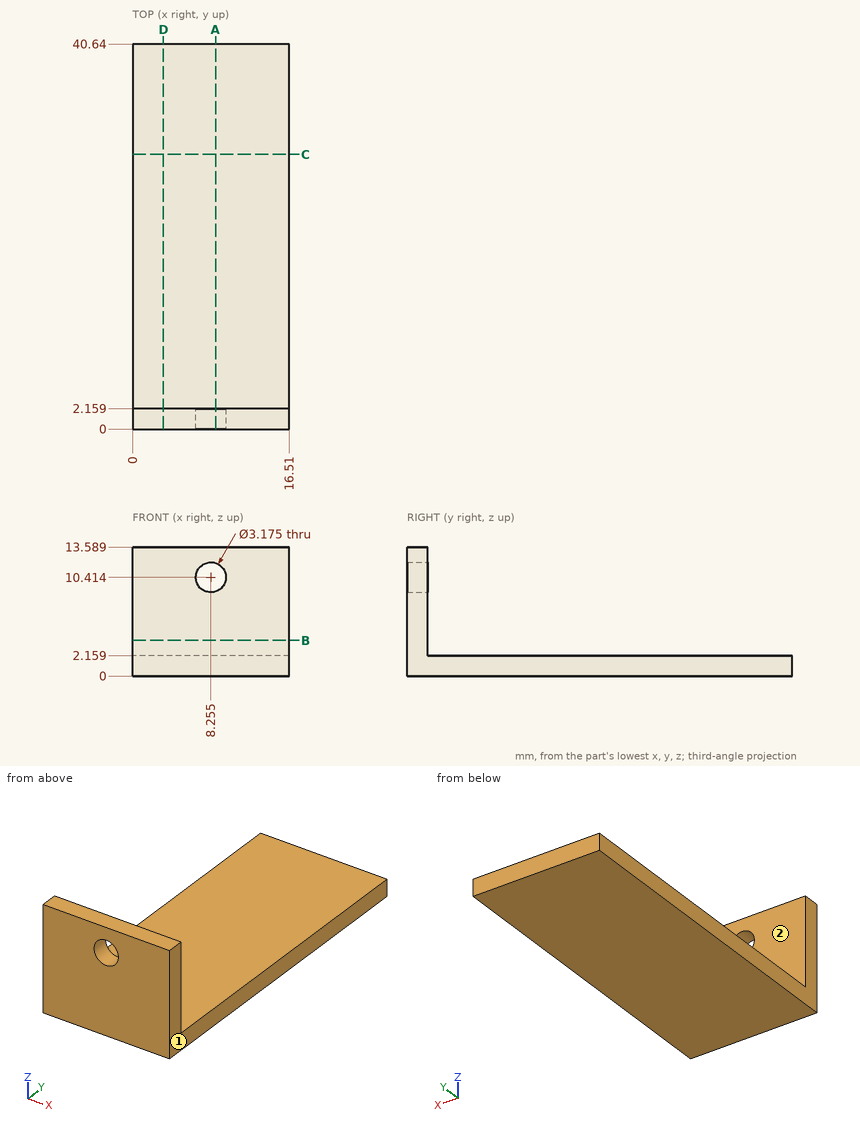
Part print with two shaded views. Sizes in mm from the minimum x, y, z corner. A direction names the side the tool comes from. Give positions to 0.01 mm unless a question says otherwise; leave off trailing zeros. Order: outer loops, then holes, each group sorted by start corner. A loop starts at its lowest first (then second) coordinate and runs counter-clockwise, first axis right, second up.
(1) Flat gauge pins, fed straight in: pin 1 (5.5 mm diameter, centred on x = 9.5, z = 5.5, fed in from +Y); pin 2 (1 mm diameter, centred on x = 7.5, y = 18.5, fed in from +Z). Where does each tip first touch, or does it go through?
(2) Saw through at B-B, the plane z = 3.75. Give the cut face in (x, y).
(3) Drill centre line: L1, parallel to Z at x = 12.5, y = 5. Where is it in solid material? Low to high.
(4) Saw through at D-D, the plane x = 3.25. Give the cut face in (y, z).
(5) Tool access for the marked faces 1 and 2: list every direction of +Z, -Z, +X, -X, +Y, -Y with a clear straight run to the whole face (end or side of a thin tool).
(6) Saw through at A-A, the plane x = 8.75. Give the cut face in (y, z), then the cut area to 3 significant figures.
Results found:
1. pin 1: stops at y = 2.16
1. pin 2: stops at z = 2.16
2. outline: (0, 0) - (16.51, 0) - (16.51, 2.16) - (0, 2.16) - close
3. L1: z = 0 to 2.16
4. outline: (0, 0) - (40.64, 0) - (40.64, 2.16) - (2.16, 2.16) - (2.16, 13.59) - (0, 13.59) - close
5. face 1: +Z, -Z, +X, +Y, -Y
5. face 2: +Z, +X, -X, +Y
6. outline: (0, 0) - (40.64, 0) - (40.64, 2.16) - (2.16, 2.16) - (2.16, 8.91) - (0, 8.91) - close; (0, 11.92) - (2.16, 11.92) - (2.16, 13.59) - (0, 13.59) - close
6. area: 106 mm2
